Verification items for this drawing (mm, ordinates from the low corner). Round coordinates to 2 decimals unless told otherwise and drop trailing zeros. Loops run counter-clockwise (first coordinate to the right, second up) from the corner with the lowest first, then second, coordinate; pieces in that order, holes last. Notation, with made-up numbers: (-27.5, 4) - (-3.5, 4) arc R13 ccw to (-3.5, 23) - close; hole circle Ø7 at (80, 1). An arc over 180 degrees is marked (long way). Answer in a Markdown table with one row per item. Add a question column.
(1) Cross-section at B-B on y = 27. Enter the section's corners in (x, z), then the cut area to 3 significant figures.
(2) Cross-section at D-D on y = 5.5. Enter the section's corners in (x, z), then the cut area to 3 significant figures.
(3) Cross-section at A-A on x = 100. Enter the section's corners in (y, z).
(4) Thickness scan on line 1 along Y through (x, z) = (112, 73.5); line 2 along X through (y, z) = (22.5, 69.5); line 3 along X through (y, z) = (16, 85). Record the ranges inside material, lowest first.
(5) Cross-section at C-C on z = 172. Enter the section's corners in (x, y).
(6) Gauge pin test, flat end, axial feed: pin 1 (6 mm diameter, centred on y = 35, z = 186.5, fed in from -X). Record the tip position at first contact, or that the pin passes through.
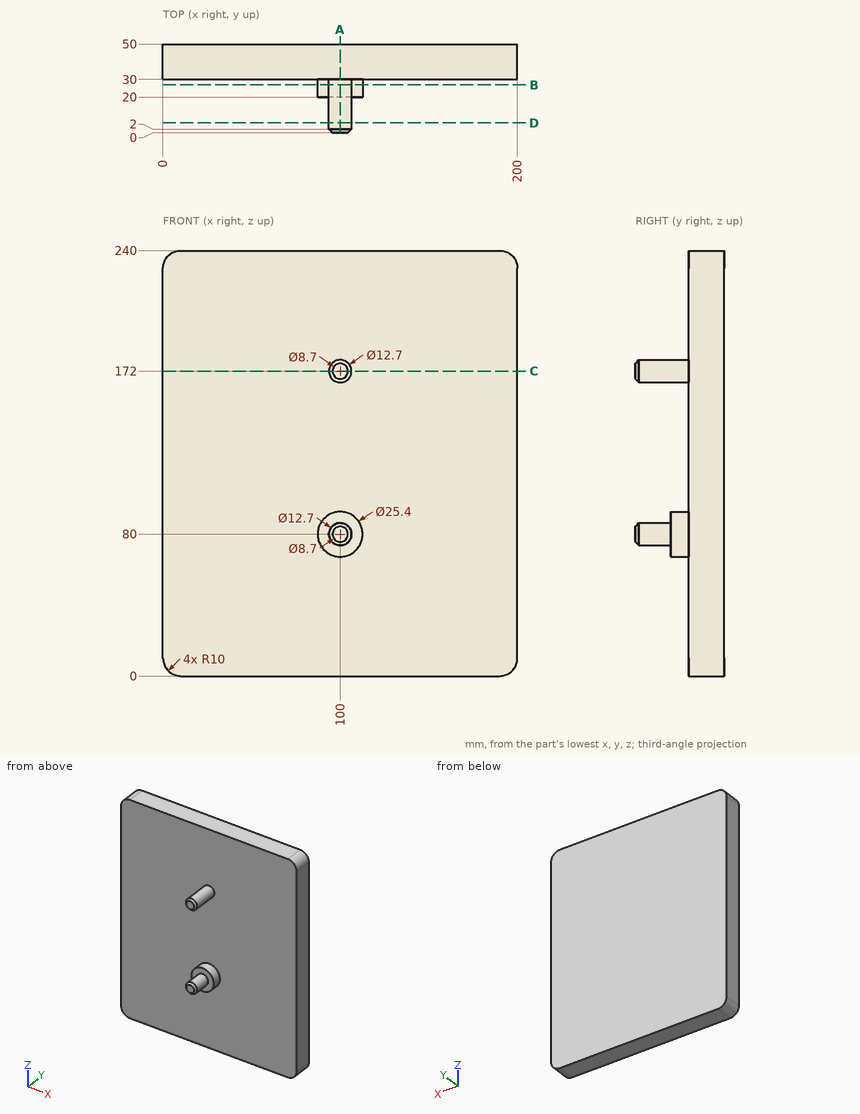
Answers:
| question | item | result |
|---|---|---|
| 1 | outline | circle Ø25.4 at (100, 80); circle Ø12.7 at (100, 172) |
| 1 | area | 633 mm^2 |
| 2 | outline | circle Ø12.7 at (100, 80); circle Ø12.7 at (100, 172) |
| 2 | area | 253 mm^2 |
| 3 | outline | (0, 75.65) - (2, 73.65) - (20, 73.65) - (20, 67.3) - (30, 67.3) - (30, 0) - (50, 0) - (50, 240) - (30, 240) - (30, 178.35) - (2, 178.35) - (0, 176.35) - (0, 167.65) - (2, 165.65) - (30, 165.65) - (30, 92.7) - (20, 92.7) - (20, 86.35) - (2, 86.35) - (0, 84.35) - close |
| 4 | line 1 | y = 30 to 50 |
| 4 | line 2 | x = 92.86 to 107.14 |
| 4 | line 3 | x = 96.09 to 103.91 |
| 5 | outline | (0, 30) - (93.65, 30) - (93.65, 2) - (95.65, 0) - (104.35, 0) - (106.35, 2) - (106.35, 30) - (200, 30) - (200, 50) - (0, 50) - close |
| 6 | pin 1 | stops at x = 0 |
